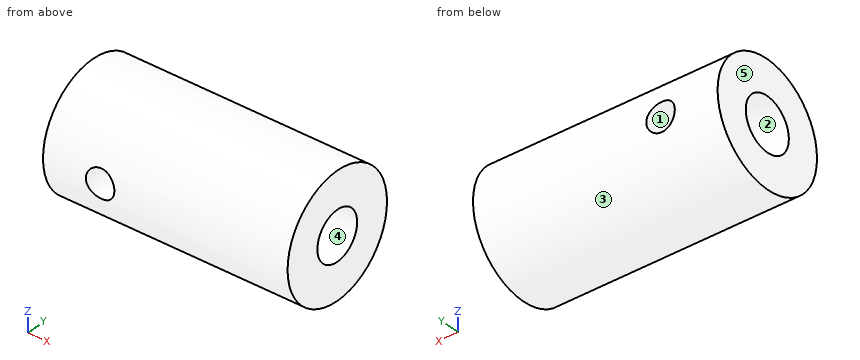
Autodesk Fusion 360 part; units mm, degrees
sketch "Sketch1" plane through (0, 0, 0) normal (1, 0, 0) x (0, 0, -1)
  circle A0 centre (0, 0) radius 3
  circle A1 centre (0, 0) radius 7.5
  dimension "d1" = 6
  dimension "d2" = 15
extrude "Extrude1" add sketch "Sketch1" against normal blind 15
sketch "Sketch2" plane through (-15, 0, 0) normal (-1, 0, 0) x (0, 0, 1)
  circle A0 centre (0, 0) radius 7.5
  circle A1 centre (0, 0) radius 3.25
  circle A2 centre (0, 0) radius 7.5
  dimension "d5" = 6.5
extrude "Extrude2" add sketch "Sketch2" along normal blind 15
sketch "Sketch3" plane through (0, 0, 0) normal (0, 1, 0) x (1, 0, 0)
  line L0 (-30, 7.5) -> (-30, -7.5)
  line L1 (0, -7.5) -> (0, 7.5)
  circle A0 centre (-23, 0) radius 1.75
  point P0 (-23, 0)
  dimension "d8" = 30
extrude "Extrude3" cut sketch "Sketch3" along normal mid plane 38
CAD build for the part. Positions are in the model's coordinates, mm. Face numbers are marked on the shaded views. A direction names the side the tool comes from. Give positions to 0.01 mm unless a question says otherwise; leave off trailing zeros. Write each loop counter-clockwise with the first axis right and the second up, starting at its lowest first coordinate (ties: lowest second). Pieces come first, ordered by that corner, then holes. Notation, with made-up numbers: (-15.5, 47) -> (-0.5, 47) arc R13 ccw to (-0.5, 57) -> close; hole circle Ø7 at (2.25, 68.25). An arc over 180 degrees is marked (long way). Write each question's results on one line, items separated by ' | '.
1. Cut at B-B, the plane z = 0. Write the cut outline in (x, y), then the cut area to 3 significant figures.
Geometry check:
outline: (-30, -7.5) -> (-24.75, -7.5) -> (-24.75, -3.25) -> (-30, -3.25) -> close; (-30, 3.25) -> (-24.75, 3.25) -> (-24.75, 7.5) -> (-30, 7.5) -> close; (-21.25, -7.5) -> (0, -7.5) -> (0, -3) -> (-15, -3) -> (-15, -3.25) -> (-21.25, -3.25) -> close; (-21.25, 3.25) -> (-15, 3.25) -> (-15, 3) -> (0, 3) -> (0, 7.5) -> (-21.25, 7.5) -> close | area: 233 mm²
2. Cut at A-A, the plane y = 0. Write the cut outline in (x, z).
Geometry check:
outline: (-30, -7.5) -> (0, -7.5) -> (0, -3) -> (-15, -3) -> (-15, -3.25) -> (-30, -3.25) -> close; (-30, 3.25) -> (-15, 3.25) -> (-15, 3) -> (0, 3) -> (0, 7.5) -> (-30, 7.5) -> close
3. Two-plate mould, pull along Y, no slides. Class the marked faces 3, 4 and 5: pulls with the +Y half, pulls with the -Y half, needs draft (parallel to the pull), parting line crosses it, or undercut.
Geometry check:
face 3: parting line crosses it | face 4: undercut | face 5: needs draft
4. Cut at D-D, the plane x = -14.5. Write the cut outline in (y, z), then the cut area to 3 significant figures.
Geometry check:
outline: circle Ø15 at (0, 0); hole circle Ø6 at (0, 0) | area: 148 mm²
5. Which spindle directions (+Z, -Z, +X, -X, +Y, -Y) get a long thin tool onto all of the face, cutting with end or side? Do the marked faces 1 and 2. Say none if no direction does.
Geometry check:
face 1: +Y, -Y | face 2: -X
6. Cut at C-C, the plane x = -23. Write the cut outline in (y, z), then the cut area to 3 significant figures.
Geometry check:
outline: (-7.29, -1.75) arc R7.5 ccw to (7.29, -1.75) -> (2.74, -1.75) arc R3.25 cw to (-2.74, -1.75) -> close; (-7.29, 1.75) -> (-2.74, 1.75) arc R3.25 cw to (2.74, 1.75) -> (7.29, 1.75) arc R7.5 ccw to start | area: 113 mm²
7. Drop flat-ended pins along their axis: P1, Ø4, axis at x = -6, y = 2.5, coming from the -Z side; P2, Ø5, axis at x = -17.5, y = 4, coming from the +Z side; P3, Ø1, axis at x = -26.5, y = -2, coming from the -Z side. Give the stop position or say it passes through.
Geometry check:
P1: z = -7.48 | P2: z = 7.35 | P3: z = -7.35
8. Wall check: probe 1 along Y at (x, z) = (-3.25, 0); probe 2 along Y at (x, z) = (-25.75, 0); probe 3 along X at (y, z) = (4.05, 0). Give the ranges that are in metal, low to high. Write a range as [from, to].
Geometry check:
probe 1: [-7.5, -3], [3, 7.5] | probe 2: [-7.5, -3.25], [3.25, 7.5] | probe 3: [-30, -24.75], [-21.25, 0]
